Build history of the part. All positions in model axes, mm. A direction names the side the tool comes from. Round coordinates to 2 decimals unless told otherwise and drop trailing zeros. Loops run counter-clockwise (first coordinate to the right, second up) from the corner with the lowest first, then second, coordinate; pieces in that order, holes last. Notation, with made-up numbers: (-33, 1) -> (4, 1) arc R19 ccw to (4, 20) -> close; hole circle Ø5 at (-19, -7). An arc over 180 degrees is marked (long way). Put each result on its own line as item: value. Start each with the question number.
```python
from build123d import *

# Parameters (mm, degrees)
F1_DEPTH = 6
F2_R     = 10
F3_R     = 3
F4_R     = 3
F5_R     = 3


with BuildPart() as f1:
    # F0 (on Front) → F1 (new body, symmetric)
    with BuildSketch(Plane.XZ):
        with BuildLine():
            Line((0, 111.17877506), (-100, 111.17877506))
            Line((-100, 111.17877506), (-100, 72.17877506))
            Line((-100, 72.17877506), (-120, 72.17877506))
            Line((-120, 72.17877506), (-120, 63.17877506))
            Line((-120, 63.17877506), (-103, 63.17877506))
            ThreePointArc((-103, 63.17877506), (-97, 57.17877506), (-103, 51.17877506))
            Line((-103, 51.17877506), (-120, 51.17877506))
            Line((-120, 51.17877506), (-120, 42.17877506))
            Line((-120, 42.17877506), (-100, 42.17877506))
            Line((-100, 42.17877506), (-100, -53.82122494))
            Line((-100, -53.82122494), (-100, -149.82122494))
            Line((-100, -149.82122494), (-120, -149.82122494))
            Line((-120, -149.82122494), (-120, -158.82122494))
            Line((-120, -158.82122494), (-103, -158.82122494))
            ThreePointArc((-103, -158.82122494), (-97, -164.82122494), (-103, -170.82122494))
            Line((-103, -170.82122494), (-120, -170.82122494))
            Line((-120, -170.82122494), (-120, -179.82122494))
            Line((-120, -179.82122494), (-100, -179.82122494))
            Line((-100, -179.82122494), (-100, -218.82122494))
            Line((-100, -218.82122494), (0, -218.82122494))
            Line((0, -218.82122494), (100, -218.82122494))
            Line((100, -218.82122494), (100, -179.82122494))
            Line((100, -179.82122494), (120, -179.82122494))
            Line((120, -179.82122494), (120, -170.82122494))
            Line((120, -170.82122494), (103, -170.82122494))
            ThreePointArc((103, -170.82122494), (97, -164.82122494), (103, -158.82122494))
            Line((103, -158.82122494), (120, -158.82122494))
            Line((120, -158.82122494), (120, -149.82122494))
            Line((120, -149.82122494), (100, -149.82122494))
            Line((100, -149.82122494), (100, -53.82122494))
            Line((100, -53.82122494), (100, 42.17877506))
            Line((100, 42.17877506), (120, 42.17877506))
            Line((120, 42.17877506), (120, 51.17877506))
            Line((120, 51.17877506), (103, 51.17877506))
            ThreePointArc((103, 51.17877506), (97, 57.17877506), (103, 63.17877506))
            Line((103, 63.17877506), (120, 63.17877506))
            Line((120, 63.17877506), (120, 72.17877506))
            Line((120, 72.17877506), (100, 72.17877506))
            Line((100, 72.17877506), (100, 111.17877506))
            Line((100, 111.17877506), (0, 111.17877506))
        make_face()
        Polygon((-75, -53.82122494), (-75, 86.17877506), (0, 86.17877506), (75, 86.17877506), (75, -53.82122494), (75, -193.82122494), (0, -193.82122494), (-75, -193.82122494), align=None, mode=Mode.SUBTRACT)
    extrude(amount=F1_DEPTH, both=True)

    # F2
    f2_edges = [f1.edges().sort_by_distance(p)[0] for p in [
        (100, 0, 111.178775),
        (-100, 0, 111.178775),
        (100, 0, -218.821225),
        (-100, 0, -218.821225),
    ]]
    fillet(f2_edges, radius=F2_R)

    # F3
    f3_edges = [f1.edges().sort_by_distance(p)[0] for p in [
        (-75, 0, -193.821225),
        (75, 0, -193.821225),
        (75, 0, 86.178775),
        (-75, 0, 86.178775),
    ]]
    fillet(f3_edges, radius=F3_R)

    # F4
    f4_edges = [f1.edges().sort_by_distance(p)[0] for p in [
        (-120, 0, -149.821225),
        (-120, 0, -179.821225),
        (120, 0, -149.821225),
        (120, 0, -179.821225),
        (120, 0, 72.178775),
        (120, 0, 42.178775),
        (-120, 0, 72.178775),
        (-120, 0, 42.178775),
    ]]
    fillet(f4_edges, radius=F4_R)

    # F5
    f5_edges = [f1.edges().sort_by_distance(p)[0] for p in [
        (100, 0, 72.178775),
        (100, 0, 42.178775),
        (100, 0, -179.821225),
        (100, 0, -149.821225),
        (-100, 0, -149.821225),
        (-100, 0, -179.821225),
        (-100, 0, 72.178775),
        (-100, 0, 42.178775),
    ]]
    fillet(f5_edges, radius=F5_R)


solid = f1.part
```
Item 1: Drop flat-ended pins along their axis: pin 1 (4 mm diameter, centred on y = -2.5, z = -51.5, fed in from +X); pin 2 (6 mm diameter, centred on x = -109.5, y = 0, fed in from +Z); pin 3 (6 mm diameter, centred on x = 112.5, y = 3, fed in from -Z). Give the stop position or say it passes through.
Item 2: 3-axis set-ups, long thin cutter, end or side, ignore diameter. For faces 4 (the face through (1, 0, -193.821)), 5 (the face through (-110, 0, 42.179)), 6 (the face through (112, 0, -170.821)): which of +Z, -Z, +X, -X, +Y, -Y reach the whole face in a straight line?
Item 3: Cut at A-A on x = -14. Write the cut outline in (y, z).
Item 4: Wall check: line 1 (Z direction, x = -108, y = 4.75); line 2 (X direction, y = 1.5, z = -55); line 3 (X direction, y = 2, z = 56.5). Give the ranges that are in metal, low to high. Write a range as from..to.
Item 5: Pull direction Z, two halves, no side cores. Call faces 1 (the face through (-81, -6, -53)), 2 (the face through (-110, 0, -179.821)), 3 (the face through (110, 0, 42.179)): +Z half, -Z half, draft (parallel to the pull), parting line (faces both ways), or undercut.
Item 6: Cut at B-B on z = -187.5. Write the cut outline in (x, y).
Ans:
1. pin 1: stops at x = 100
1. pin 2: stops at z = 72.18
1. pin 3: stops at z = -179.82
2. face 4: +Y, -Y
2. face 5: -X, +Y, -Y
2. face 6: +X, +Y, -Y
3. outline: (-6, -218.82) -> (6, -218.82) -> (6, -193.82) -> (-6, -193.82) -> close; (-6, 86.18) -> (6, 86.18) -> (6, 111.18) -> (-6, 111.18) -> close
4. line 1: z = -179.82..-170.82, -158.82..-149.82, 42.18..51.18, 63.18..72.18
4. line 2: x = -100..-75, 75..100
4. line 3: x = -97.04..-75, 75..97.04
5. face 1: draft
5. face 2: -Z half
5. face 3: undercut
6. outline: (-100, -6) -> (-75, -6) -> (-75, 6) -> (-100, 6) -> close; (75, -6) -> (100, -6) -> (100, 6) -> (75, 6) -> close
